Could you check a few things on this model? Use its own coordinates, in mm. A direction names the side the tool comes from. Round coordinates to 2 decimals unless told otherwise and drop trailing zeros. Loops run counter-clockwise (first coordinate to the right, second up) from the corner with the lowest first, then second, coordinate; pieces in that order, holes last. Notation, with made-up numbers: M 42,24.25 L 51,24.25 A22 cw 51,34.25 Z; hole C -14.75,50.25 d9. An arc over 180 degrees is marked long. Answer in a Markdown table with one row per item.
```python
from build123d import *

# Parameters (mm, degrees)
F0_W        = 72
F0_H        = 23.5
F0_R        = 2
F0_W_2      = 44
F0_H_2      = 15.5
F1_DEPTH    = 2
F2_DEPTH    = 8
F3_T1_DEPTH = 193.9586602962


# Not quite as in the source:
# - a fillet or chamfer that OpenCascade refuses, or shapes differently, is made with other operations: its cross-section is extruded or revolved along the edge and cut away or added


with BuildPart() as f1:
    # F0 (on Top) → F1 (new body)
    with BuildSketch(Plane.XY):
        with Locations((36, -11.75)):
            Rectangle(F0_W, F0_H)
        with Locations((6, -11.75)):
            Circle(F0_R, mode=Mode.SUBTRACT)
        with Locations((36, -11.75)):
            Rectangle(F0_W_2, F0_H_2, mode=Mode.SUBTRACT)
        with Locations((66, -11.75)):
            Circle(F0_R, mode=Mode.SUBTRACT)
    extrude(amount=F1_DEPTH)

    # F2 (add): a face of the model
    f2_faces = [f1.faces().sort_by_distance(p)[0] for p in [
        (36, -0.7573803536, 2),
    ]]
    extrude(f2_faces, amount=F2_DEPTH)

    # F3: chamfer of 23.5 x 8 on 1 edges, made by hand

    # F3_s2 → F3_t1 (cut)
    with BuildSketch(Plane.YZ.offset(-60.9793301481)):
        Polygon((-23.5, 2), (0, 10), (-23.5, 10), align=None)
    extrude(amount=F3_T1_DEPTH, mode=Mode.SUBTRACT)


solid = f1.part
```
1) I need wall thicknesses on line 1 (X direction, y = -11.75, z = 3); line 2 (Y direction, x = 28.5, z = 0.5); line 3 (Y direction, x = 6, z = 1.5). Which ranges of each line are inside material? Lowest first, please.
Computed:
| item | result |
|---|---|
| line 1 | x = 0 to 4, 8 to 14, 58 to 64, 68 to 72 |
| line 2 | y = -23.5 to -19.5, -4 to 0 |
| line 3 | y = -23.5 to -13.75, -9.75 to 0 |
2) I want a section at B-B, the plane x = 26. Please give me the cut outline in (y, z), plus the area to 3 significant figures.
Computed:
| item | result |
|---|---|
| outline | M -23.5,0 L -19.5,0 L -19.5,3.36 L -23.5,2 Z; M -4,0 L 0,0 L 0,10 L -4,8.64 Z |
| area | 48.0 mm² |
3) I want a section at C-C, the plane y = -17. Please give me the cut outline in (x, z).
Computed:
| item | result |
|---|---|
| outline | M 0,0 L 14,0 L 14,4.21 L 0,4.21 Z; M 58,0 L 72,0 L 72,4.21 L 58,4.21 Z |
4) I want a section at A-A, the plane y = -11.75. Please give me the cut outline in (x, z), plus the area to 3 significant figures.
Computed:
| item | result |
|---|---|
| outline | M 0,0 L 4,0 L 4,6 L 0,6 Z; M 8,0 L 14,0 L 14,6 L 8,6 Z; M 58,0 L 64,0 L 64,6 L 58,6 Z; M 68,0 L 72,0 L 72,6 L 68,6 Z |
| area | 120 mm² |
5) Will these pins go through, and if not, where does the flat tip stop? P1, Ø8, axis at x = 39.5, y = -18.5, coming from the +Z side; P2, Ø6.5, axis at x = 6, y = -11.75, coming from the +Z side; P3, Ø2.5, axis at x = 38, z = 5.5, coming from the -Y side.
Computed:
| item | result |
|---|---|
| P1 | stops at z = 3.36 |
| P2 | stops at z = 7.11 |
| P3 | stops at y = -4 |
6) I want a section at D-D, the plane z = 5. Please give me the cut outline in (x, y), plus the area to 3 significant figures.
Computed:
| item | result |
|---|---|
| outline | M 0,-14.69 L 14,-14.69 L 14,-4 L 58,-4 L 58,-14.69 L 72,-14.69 L 72,0 L 0,0 Z; hole C 6,-11.75 d4; hole C 66,-11.75 d4 |
| area | 562 mm² |
7) Which directions (+Z, -Z, +X, -X, +Y, -Y) give clear straight access to the entire face, cutting with the end or side of a thin tool? Please do faces 4 (the face through (0, -9, 4)), 5 (the face through (58, -10, 3)).
Computed:
| item | result |
|---|---|
| face 4 | +Z, -Z, -X, +Y, -Y |
| face 5 | +Z, -Z |
8) If we mould it in two halves opening along X, with no side actions, what happens to faces 1 (the face through (36, -19.5, 2)), 2 (the face through (72, -9, 4)), 3 (the face through (35, 0, 5))? For each: released by +X, released by -X, zero draft, split by the parting line, or undercut.
Computed:
| item | result |
|---|---|
| face 1 | undercut |
| face 2 | released by +X |
| face 3 | zero draft |
